Answer from the drawing. Dimensions are ordinates in mm from the lowest x, y and z of the part. A direction names the side the tool comes from. Coordinates: 2 decimals unless noted, no trailing zeros. Order: outer loops, then holes, each group sorted by start corner. A loop starts at its lowest first (then second) coordinate and runs counter-clockwise, first axis right, second up.
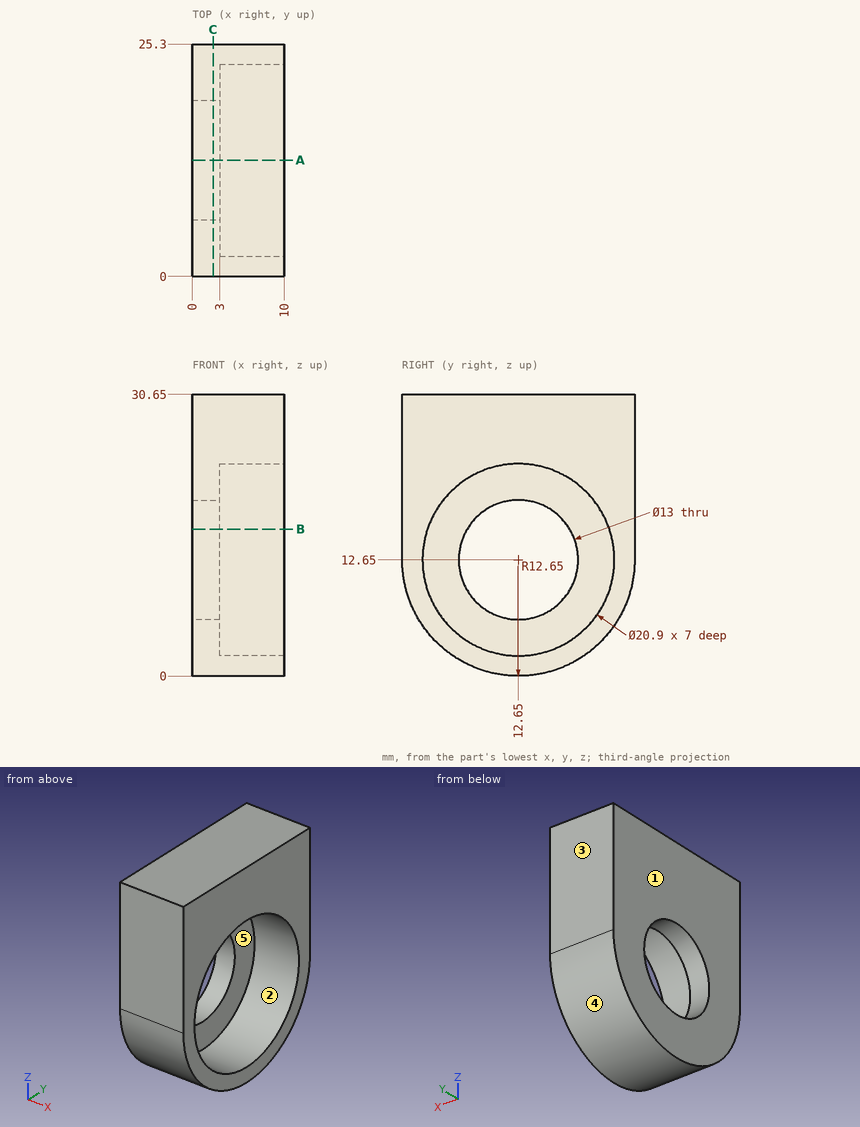
1. The part is cut by section A-A (y = 12.65). Determine the outline of the cut face in (x, z), plus the area to 3 significant figures.
2. The part is cut by section C-C (x = 2.25). Determine the outline of the cut face in (y, z), plus the area to 3 significant figures.
3. The part is cut by section B-B (z = 16). Determine the outline of the cut face in (x, y), plus the area to 3 significant figures.
4. Flat-ended cylindrical pins translate along their axes: pin 1 (1.5 mm diameter, centred on y = 5, z = 25, fed in from -X); pin 2 (1 mm diameter, centred on x = 1.5, z = 10, fed in from +Y); pin 3 (5 mm diameter, centred on x = 1, y = 18, fed in from -Z); pin 4 (5 mm diameter, centred on x = 2, y = 20, fed in from -Z). Find the tip coordinate at first contact, or state that the pin passes through.
5. Consider probe 1 along Y at (x, z) = (0.7, 12.65); probe 2 along Y at (x, z) = (6.25, 12.65); probe 3 along X at (y, z) = (20.25, 12). Determine where each line is inside the solid, lowest interval first.
6. For the marked faces 1 and 2, determine the directions among +Z, -Z, +X, -X, +Y, -Y from which every point of the face is accessible in a straight line to the end or side of a thin tool.
7. The mould has two halves that part along Z. Classify the marked faces 3, 4 and 5: released by +Z, released by -Z, zero draft, split by the parting line, or undercut.
Worked out:
1. outline: (0, 0) - (10, 0) - (10, 2.2) - (3, 2.2) - (3, 6.15) - (0, 6.15) - close; (0, 19.15) - (3, 19.15) - (3, 23.1) - (10, 23.1) - (10, 30.65) - (0, 30.65) - close
1. area: 121 mm2
2. outline: (0, 12.65) arc R12.65 ccw to (25.3, 12.65) - (25.3, 30.65) - (0, 30.65) - close; hole circle Ø13 at (12.65, 12.65)
2. area: 574 mm2
3. outline: (0, 0) - (10, 0) - (10, 2.75) - (3, 2.75) - (3, 7.08) - (0, 7.08) - close; (0, 18.22) - (3, 18.22) - (3, 22.55) - (10, 22.55) - (10, 25.3) - (0, 25.3) - close
3. area: 81.0 mm2
4. pin 1: stops at x = 0
4. pin 2: stops at y = 25.12
4. pin 3: stops at z = 0.33
4. pin 4: stops at z = 0.97
5. probe 1: y = 0 to 6.15, 19.15 to 25.3
5. probe 2: y = 0 to 2.2, 23.1 to 25.3
5. probe 3: x = 0 to 3
6. face 1: +Z, -Z, -X, +Y, -Y
6. face 2: +X
7. face 3: zero draft
7. face 4: released by -Z
7. face 5: undercut
